```python
from build123d import *

# Parameters (mm, degrees)
F1_DEPTH = 76.4
F2_R     = 5


with BuildPart() as f1:
    # F0 (on Front) → F1 (new body, symmetric)
    with BuildSketch(Plane.XZ):
        Polygon((23.964551, 12.702267), (-23.207255, 12.520527), (0.53604, -28.240586), align=None)
    extrude(amount=F1_DEPTH, both=True)

    # F2
    f2_edges = [f1.edges().sort_by_distance(p)[0] for p in [
        (0.378648, -76.4, 12.611397),
        (-11.335608, -76.4, -7.860029),
        (12.250295, -76.4, -7.769159),
        (0.378648, 76.4, 12.611397),
        (-11.335608, 76.4, -7.860029),
        (12.250295, 76.4, -7.769159),
        (-23.207255, 0, 12.520527),
        (0.53604, 0, -28.240586),
        (23.964551, 0, 12.702267),
    ]]
    fillet(f2_edges, radius=F2_R)


solid = f1.part
```
Input: part model. Units: mm. Frame: model coordinates. Give positions to 0.01 mm unless a question says otherwise; leave off trailing zeros. Order: outer loops, then holes, each group sorted by start corner. A loop starts at its lowest first (then second) coordinate and runs counter-clockwise, first axis right, second up.
1. Pin query (flat end, axial travel): pin 1 (1.5 mm diameter, centred on x = 9, y = -48.5, fed in from +Z); pin 2 (1.5 mm diameter, centred on y = -54.5, z = -14.5, fed in from -X); pin 3 (6 mm diameter, centred on x = -3, y = 49, fed in from -Z). Return the tip coordinate at first contact, or that it passes through.
Derived:
pin 1: stops at z = 12.65
pin 2: stops at x = -7.9
pin 3: stops at z = -23.22
2. Material intervals for L1, parallel to X at y = 3.5, z = -8; L2, parallel to Y at x = -9.5, z = 10.5; L3, parallel to Z at x = 16, y = 32.5, sorted ascending.
Derived:
L1: x = -11.25 to 12.12
L2: y = -75.45 to 75.45
L3: z = -1.22 to 12.62
3. Section A-A on y = 36. Return the cut outline in (x, z), and give its area (3 significant figures).
Derived:
outline: (-18.85, 5.04) - (-3.82, -20.76) arc R5 ccw to (4.84, -20.72) - (19.66, 5.19) arc R5 ccw to (15.3, 12.67) - (-14.55, 12.55) arc R5 ccw to start
area: 912 mm2
